Input: part model. Units: mm. Frame: model coordinates. A direction names the side the tool comes from. Round coordinates to 2 decimals unless told otherwise and drop trailing zeros. Order: outer loops, then holes, each group sorted by start corner. A loop starts at its lowest first (then second) coordinate and runs counter-clockwise, first axis right, second up. Notation, with made-up numbers: (31.25, 81.5) -> (63.25, 81.5) arc R28 cw to (63.25, 116.5) -> close; hole circle Ø9 at (-2.5, -15). An arc over 180 degrees is marked (long way). Use a Markdown table: item, result.
from build123d import *

# Parameters (mm, degrees)
ESQUISSE1_W        = 45
ESQUISSE1_H        = 57
ESQUISSE1_W_2      = 23
ESQUISSE1_H_2      = 43
BOSS_EXTRU_1_DEPTH = 2
ESQUISSE2_W        = 45
ESQUISSE2_H        = 57
ESQUISSE2_W_2      = 41
ESQUISSE2_H_2      = 53
BOSS_EXTRU_2_DEPTH = 45
ESQUISSE3_W        = 9
ESQUISSE3_H        = 10
ESQUISSE3_R        = 2.5
BOSS_EXTRU_3_DEPTH = 4


with BuildPart() as part:
    # Esquisse1 → Boss.-Extru.1 (new body)
    with BuildSketch(Plane(origin=(0, 0, 0), x_dir=(1, 0, 0), z_dir=(0, 1, 0))):
        with Locations((11.5, 21.5)):
            Rectangle(ESQUISSE1_W, ESQUISSE1_H)
        with Locations((11.5, 21.5)):
            Rectangle(ESQUISSE1_W_2, ESQUISSE1_H_2, mode=Mode.SUBTRACT)
    extrude(amount=BOSS_EXTRU_1_DEPTH)

    # Esquisse2 → Boss.-Extru.2 (add)
    with BuildSketch(Plane(origin=(0, 2, 0), x_dir=(1, 0, 0), z_dir=(0, 1, 0))):
        with Locations((11.5, 21.5)):
            Rectangle(ESQUISSE2_W, ESQUISSE2_H)
        with Locations((11.5, 21.5)):
            Rectangle(ESQUISSE2_W_2, ESQUISSE2_H_2, mode=Mode.SUBTRACT)
    extrude(amount=BOSS_EXTRU_2_DEPTH)

    # Esquisse3 → Boss.-Extru.3 (add)
    with BuildSketch(Plane(origin=(0, 47, 0), x_dir=(1, 0, 0), z_dir=(0, 1, 0))):
        with Locations((-4.5, 21.5)):
            Rectangle(ESQUISSE3_W, ESQUISSE3_H)
        with Locations((-4.5, 21.5)):
            Circle(ESQUISSE3_R, mode=Mode.SUBTRACT)
        with Locations((27.5, 21.5)):
            Rectangle(ESQUISSE3_W, ESQUISSE3_H)
        with Locations((27.5, 21.5)):
            Circle(ESQUISSE3_R, mode=Mode.SUBTRACT)
    extrude(amount=-BOSS_EXTRU_3_DEPTH)


solid = part.part
1) Cut plane D-D on y = 23. Return loops of the section in (x, z).
Results found:
| item | result |
|---|---|
| outline | (-11, -50) -> (34, -50) -> (34, 7) -> (-11, 7) -> close; hole (-9, -48) -> (32, -48) -> (32, 5) -> (-9, 5) -> close |
2) Line query: L1, parallel to X at y = 43.95, z = -21.5; L2, parallel to Z at x = -4.5, y = 45.65; L3, parallel to X at y = 10, z = -40.5. Output: solid intervals per line, ascending. Write a range as [from, to].
Results found:
| item | result |
|---|---|
| L1 | x = [-11, -7], [-2, 0], [23, 25], [30, 34] |
| L2 | z = [-50, -48], [-26.5, -24], [-19, -16.5], [5, 7] |
| L3 | x = [-11, -9], [32, 34] |
3) Cut plane C-C on z = -21.5. Return loops of the section in (x, y).
Results found:
| item | result |
|---|---|
| outline | (-11, 0) -> (0, 0) -> (0, 2) -> (-9, 2) -> (-9, 43) -> (-7, 43) -> (-7, 47) -> (-11, 47) -> close; (-2, 43) -> (0, 43) -> (0, 47) -> (-2, 47) -> close; (23, 0) -> (34, 0) -> (34, 47) -> (30, 47) -> (30, 43) -> (32, 43) -> (32, 2) -> (23, 2) -> close; (23, 43) -> (25, 43) -> (25, 47) -> (23, 47) -> close |
4) Cut plane B-B on x = 6.5. Return loops of the section in (y, z), and give its area (3 significant figures).
Results found:
| item | result |
|---|---|
| outline | (0, -50) -> (47, -50) -> (47, -48) -> (2, -48) -> (2, -43) -> (0, -43) -> close; (0, 0) -> (2, 0) -> (2, 5) -> (47, 5) -> (47, 7) -> (0, 7) -> close |
| area | 208 mm² |
5) Cut plane A-A on z = -28. Return loops of the section in (x, y), and give its area (3 significant figures).
Results found:
| item | result |
|---|---|
| outline | (-11, 0) -> (0, 0) -> (0, 2) -> (-9, 2) -> (-9, 47) -> (-11, 47) -> close; (23, 0) -> (34, 0) -> (34, 47) -> (32, 47) -> (32, 2) -> (23, 2) -> close |
| area | 224 mm² |
6) Pin query (flat end, axial travel): pin 1 Ø8 at (x, z) = (5.5, -2.5) entering from +Y. Return the tip coordinate at first contact, or that it passes through.
Results found:
| item | result |
|---|---|
| pin 1 | stops at y = 2 |
7) Set-up query: faces 4 (the flat face through (11, 23, -50)), 5 (the flat face through (-0.3, 47, -21.6)), 6 (the flat face through (-5, 45, -26.5)), 7 (the flat face through (-6, 43, -24)), 8 (the flat face through (23, 1, -21)). Return all of +Z, -Z, +X, -X, +Y, -Y with unobstructed straight access to the full face (end or side cutting, diameter ignored); none if empty.
Results found:
| item | result |
|---|---|
| face 4 | -Z, +X, -X, +Y, -Y |
| face 5 | +Z, -Z, +X, -X, +Y |
| face 6 | +Y |
| face 7 | none |
| face 8 | +Y, -Y |
8) Pull-direction query (Y, two-part tool) for faces 1 (the flat face through (26, 43, -24)), 2 (the flat face through (23, 45, -21)), 3 (the flat face through (26, 0, -22)); classes: +Y half, -Y half, draft (parallel to the pull), parting line (faces both ways), or undercut.
Results found:
| item | result |
|---|---|
| face 1 | undercut |
| face 2 | draft |
| face 3 | -Y half |
